```python
from build123d import *

# Parameters (mm, degrees)
SKETCH_1_W          = 73
SKETCH_1_H          = 34
EXTRUDE_1_DEPTH     = 2
SKETCH_2_R          = 4
SKETCH_2_W          = 12
SKETCH_2_H          = 5
CUT_EXTRUDE_1_DEPTH = 2
SKETCH_3_W          = 8
SKETCH_3_H          = 6
EXTRUDE_2_DEPTH     = 2
SKETCH_4_R          = 1.1
CUT_EXTRUDE_2_DEPTH = 2
FILLET_1_R          = 0.4
CHAMFER_1_SIZE      = 0.2


with BuildPart() as part:
    # 草图1 → 凸台-拉伸1 (new body)
    with BuildSketch(Plane(origin=(0, 0, 0), x_dir=(0, 0, -1), z_dir=(1, 0, 0))):
        with Locations((36.5, 17)):
            Rectangle(SKETCH_1_W, SKETCH_1_H)
    extrude(amount=EXTRUDE_1_DEPTH)

    # 草图2 → 切除-拉伸1 (cut)
    with BuildSketch(Plane(origin=(2, 0, 0), x_dir=(0, 0, -1), z_dir=(1, 0, 0))):
        with Locations((22.5, 25.4)):
            Circle(SKETCH_2_R)
        with Locations((52.5, 26.5)):
            Rectangle(SKETCH_2_W, SKETCH_2_H)
    extrude(amount=-CUT_EXTRUDE_1_DEPTH, mode=Mode.SUBTRACT)

    # 草图3 → 凸台-拉伸2 (add)
    with BuildSketch(Plane.ZY):
        with Locations((-69, 37)):
            Rectangle(SKETCH_3_W, SKETCH_3_H)
        with Locations((-4, 37)):
            Rectangle(SKETCH_3_W, SKETCH_3_H)
    extrude(amount=-EXTRUDE_2_DEPTH)

    # 草图4 → 切除-拉伸2 (cut)
    with BuildSketch(Plane(origin=(2, 0, 0), x_dir=(0, 0, -1), z_dir=(1, 0, 0))):
        with Locations((4, 36)):
            Circle(SKETCH_4_R)
        with Locations((69, 36)):
            Circle(SKETCH_4_R)
        with Locations((69, 4)):
            Circle(SKETCH_4_R)
        with Locations((4, 4)):
            Circle(SKETCH_4_R)
    extrude(amount=-CUT_EXTRUDE_2_DEPTH, mode=Mode.SUBTRACT)

    # 圆角1
    fillet_1_edges = [part.edges().sort_by_distance(p)[0] for p in [
        (1, 40, -73),
        (1, 40, -65),
        (1, 34, -65),
        (1, 40, 0),
        (1, 34, -8),
        (1, 40, -8),
        (1, 0, -73),
        (1, 0, 0),
    ]]
    fillet(fillet_1_edges, radius=FILLET_1_R)

    # 倒角1
    chamfer_1_edges = [part.edges().sort_by_distance(p)[0] for p in [
        (2, 0.117157288, -72.882842712),
        (2, 39.882842712, -72.882842712),
        (2, 39.882842712, -65.117157288),
        (2, 39.882842712, -7.882842712),
        (2, 39.882842712, -0.117157288),
        (0, 34.117157288, -8.117157288),
        (2, 34.117157288, -8.117157288),
        (0, 34.117157288, -64.882842712),
        (2, 34.117157288, -64.882842712),
        (0, 26.5, -46.5),
        (0, 29, -52.5),
        (0, 26.5, -58.5),
        (0, 24, -52.5),
        (2, 26.5, -46.5),
        (2, 24, -52.5),
        (2, 26.5, -58.5),
        (2, 29, -52.5),
        (0, 25.4, -18.5),
        (2, 25.4, -18.5),
        (0, 4, -2.9),
        (2, 4, -2.9),
        (0, 4, -67.9),
        (2, 4, -67.9),
        (0, 36, -67.9),
        (2, 36, -67.9),
        (0, 36, -2.9),
        (2, 36, -2.9),
        (0, 20, 0),
        (2, 20, 0),
        (0, 40, -4),
        (0, 37, -8),
        (0, 34, -36.5),
        (0, 37, -65),
        (0, 40, -69),
        (0, 20, -73),
        (0, 0, -36.5),
        (0, 0.117157288, -0.117157288),
        (0, 0.117157288, -72.882842712),
        (0, 39.882842712, -72.882842712),
        (0, 39.882842712, -65.117157288),
        (0, 39.882842712, -7.882842712),
        (0, 39.882842712, -0.117157288),
        (2, 40, -4),
        (2, 0, -36.5),
        (2, 20, -73),
        (2, 40, -69),
        (2, 37, -65),
        (2, 34, -36.5),
        (2, 37, -8),
        (2, 0.117157288, -0.117157288),
    ]]
    chamfer(chamfer_1_edges, length=CHAMFER_1_SIZE)


solid = part.part
```
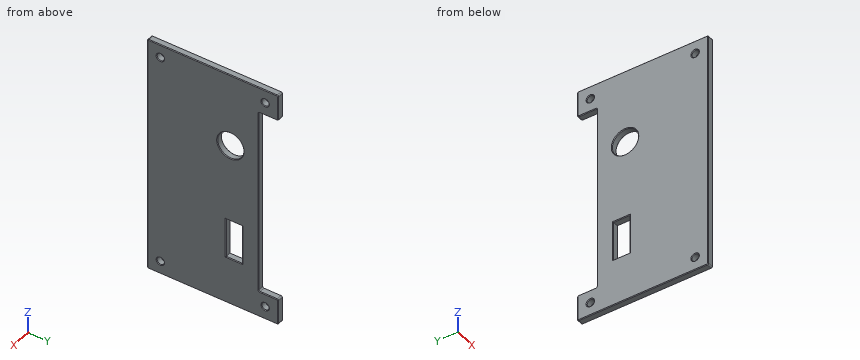
Can you work these out from the model? Positions are in its coordinate system, mm. Round coordinates to 2 decimals unless told otherwise and drop trailing zeros. Order: outer loops, then holes, each group sorted by start corner. A loop starts at its lowest first (then second) coordinate and runs counter-clockwise, first axis right, second up. Notation, with made-up numbers: (38.5, -35) -> (43.5, -35) arc R31 cw to (43.5, -11) -> close; hole circle Ø3 at (12, 74.25). An arc over 180 degrees is marked (long way). Return JSON: item names as keys, results as strings. Group by question number.
1. If we section it at B-B, the plane z = -4: Write out the boundary of the cut face in (x, y).
2. If we section it at A-A, the plane z = -22.5: Write out the boundary of the cut face in (x, y), then the cut area to 3 significant figures.
3. I need wall thicknesses on line 1 (Y direction, x = 1.15, z = -4); line 2 (Z direction, x = 1.3, y = 26.5); line 3 (Y direction, x = 1.3, z = -22.5). Which ranges of each line are inside material? Lowest first, please. Write a range as [from, to].
4. If we section it at D-D, the plane x = 1.1: Write out the boundary of the cut face in (y, z).
5. Will these pins go through, and if not, where does the flat tip stop? pin 1 (2 mm diameter, centred on y = 4, z = -4, fed in from -X); pin 2 (1 mm diameter, centred on x = 1, z = -58.5, fed in from +Y).
6. If we section it at C-C, the plane y = 36: Count the separate pieces of the cut face and the enclosed holes in it, then the cut area to 3 significant figures.
Output values:
{
 "1": {"outline": "(0, 0.2) -> (0.2, 0) -> (1.8, 0) -> (2, 0.2) -> (2, 2.7) -> (1.8, 2.9) -> (0.2, 2.9) -> (0, 2.7) -> close; (0, 5.3) -> (0.2, 5.1) -> (1.8, 5.1) -> (2, 5.3) -> (2, 34.7) -> (1.8, 34.9) -> (0.2, 34.9) -> (0, 34.7) -> close; (0, 37.3) -> (0.2, 37.1) -> (1.8, 37.1) -> (2, 37.3) -> (2, 39.8) -> (1.8, 40) -> (0.2, 40) -> (0, 39.8) -> close"},
 "2": {"outline": "(0, 0.2) -> (0.2, 0) -> (1.8, 0) -> (2, 0.2) -> (2, 21.2) -> (1.8, 21.4) -> (0.2, 21.4) -> (0, 21.2) -> close; (0, 29.6) -> (0.2, 29.4) -> (1.8, 29.4) -> (2, 29.6) -> (2, 33.8) -> (1.8, 34) -> (0.2, 34) -> (0, 33.8) -> close", "area": "51.8 mm²"},
 "3": {"line 1": "[0, 2.9], [5.1, 34.9], [37.1, 40]", "line 2": "[-73, -58.5], [-46.5, -26.35], [-18.65, 0]", "line 3": "[0, 21.4], [29.4, 34]"},
 "4": {"outline": "(0, -72.6) arc R0.4 ccw to (0.4, -73) -> (39.6, -73) arc R0.4 ccw to (40, -72.6) -> (40, -65.4) arc R0.4 ccw to (39.6, -65) -> (34.4, -65) arc R0.4 cw to (34, -64.6) -> (34, -8.4) arc R0.4 cw to (34.4, -8) -> (39.6, -8) arc R0.4 ccw to (40, -7.6) -> (40, -0.4) arc R0.4 ccw to (39.6, 0) -> (0.4, 0) arc R0.4 ccw to (0, -0.4) -> close; hole circle Ø2.2 at (4, -69); hole circle Ø2.2 at (4, -4); hole circle Ø8 at (25.4, -22.5); hole (24, -58.5) -> (29, -58.5) -> (29, -46.5) -> (24, -46.5) -> close; hole circle Ø2.2 at (36, -69); hole circle Ø2.2 at (36, -4)"},
 "5": {"pin 1": "through", "pin 2": "y = 34"},
 "6": {"separate pieces": "4", "enclosed holes": "0", "area": "22.9 mm²"}
}
